```python
from build123d import *

# Parameters (mm, degrees)
BOSS_EXTRUDE1_DEPTH = 25
SKETCH5_R           = 8
BOSS_EXTRUDE2_DEPTH = 35
SKETCH6_R           = 8
BOSS_EXTRUDE3_DEPTH = 35
CUT_EXTRUDE1_DEPTH  = 35
SKETCH9_R           = 5.1
CUT_EXTRUDE2_DEPTH  = 17
SKETCH10_R          = 5.1
CUT_EXTRUDE3_DEPTH  = 17
SKETCH11_R          = 0.5
CUT_EXTRUDE4_DEPTH  = 49.48192396
CUT_EXTRUDE5_REACH  = 44.001
SKETCH12_R          = 1.6
CUT_EXTRUDE7_DEPTH  = 66.003822587


# Read off the part's stored shape, not the designer's step: Mirror1
with BuildPart() as part:
    # Sketch3 → Boss-Extrude1 (new body)
    with BuildSketch(Plane(origin=(0, 0, 0), x_dir=(-0.9678879191476432, 0.2513821313618881, 0), z_dir=(0, 0, 1))):
        Polygon((-6.013757892, -13.576992157), (13.576992157, -6.013757892), (6.013757892, 13.576992157), (-13.576992157, 6.013757892), align=None)
    extrude(amount=BOSS_EXTRUDE1_DEPTH)

    # Sketch5 → Boss-Extrude2 (add)
    with BuildSketch(Plane(origin=(0, 0, 0), x_dir=(-0.6605627762289513, -0.729230336843708, -0.17854952950795708), z_dir=(0.5774000057119382, -0.6454527352206789, 0.499999999999998))):
        with Locations(Location((0, 0, 0), (0, 0, 168.101929209))):
            Circle(SKETCH5_R)
    extrude(amount=BOSS_EXTRUDE2_DEPTH)

    # Sketch6 → Boss-Extrude3 (add)
    with BuildSketch(Plane(origin=(0, 0, 0), x_dir=(-0.7035639492311271, 0.6172392366079582, 0.3521554970945721), z_dir=(-0.4160720061092846, -0.7595288577349762, 0.499999999999998))):
        with Locations(Location((0, 0, 0), (0, 0, 312.286757046))):
            Circle(SKETCH6_R)
    extrude(amount=BOSS_EXTRUDE3_DEPTH)

    # Sketch8 → Cut-Extrude1 (cut)
    with BuildSketch(Plane(origin=(0, 0, 0), x_dir=(-0.9678879191476432, 0.2513821313618881, 0), z_dir=(0, 0, 1))):
        Polygon((-36.845563498, -70.986857451), (-76.079837432, 33.240527854), (43.363854901, 78.202670298), (82.598128835, -26.024715007), align=None)
    extrude(amount=-CUT_EXTRUDE1_DEPTH, mode=Mode.SUBTRACT)

    # Sketch9 → Cut-Extrude2 (cut)
    with BuildSketch(Plane(origin=(20.2090002, -22.590845733, 17.5), x_dir=(0.6605627762289512, 0.7292303368437081, 0.1785495295079571), z_dir=(0.5774000057119382, -0.6454527352206788, 0.499999999999998))):
        with Locations(Location((0, 0, 0), (0, 0, 348.101929209))):
            Circle(SKETCH9_R)
    extrude(amount=-CUT_EXTRUDE2_DEPTH, mode=Mode.SUBTRACT)

    # Sketch10 → Cut-Extrude3 (cut)
    with BuildSketch(Plane(origin=(-14.562520214, -26.583510021, 17.5), x_dir=(-0.7035639492311272, 0.6172392366079582, 0.352155497094572), z_dir=(-0.41607200610928446, -0.7595288577349761, 0.499999999999998))):
        with Locations(Location((0, 0, 0), (0, 0, 129.311285717))):
            Circle(SKETCH10_R)
    extrude(amount=-CUT_EXTRUDE3_DEPTH, mode=Mode.SUBTRACT)

    # Sketch11 → Cut-Extrude4 (cut, through all)
    with BuildSketch(Plane(origin=(0, 0, 25), x_dir=(0.967887919147643, -0.25138213136188803, 0), z_dir=(0, 0, 1))):
        with BuildLine():
            ThreePointArc((-3.837479182, -9.792532706), (-3.837482303, -9.790766245), (-3.837491664, -9.788999807))
            Line((-3.837491664, -9.788999807), (-4.438726063, -10.021113258))
            Line((-4.438726063, -10.021113258), (-4.670839514, -9.419878859))
            ThreePointArc((-4.670839514, -9.419878859), (-4.541586794, -10.248975564), (-3.837479182, -9.792532706))
        make_face()
        with BuildLine():
            Line((-4.438726063, -10.021113258), (-3.837491664, -9.788999807))
            ThreePointArc((-3.837491664, -9.788999807), (-4.134985421, -9.3353716), (-4.670839514, -9.419878859))
            Line((-4.670839514, -9.419878859), (-4.438726063, -10.021113258))
        make_face()
        with BuildLine():
            Line((9.419878859, -4.670839514), (10.021113258, -4.438726063))
            Line((10.021113258, -4.438726063), (9.788999807, -3.837491664))
            ThreePointArc((9.788999807, -3.837491664), (9.3353716, -4.134985421), (9.419878859, -4.670839514))
        make_face()
        with BuildLine():
            Line((9.788999807, -3.837491664), (10.021113258, -4.438726063))
            Line((10.021113258, -4.438726063), (9.419878859, -4.670839514))
            ThreePointArc((9.419878859, -4.670839514), (9.97096067, -4.804558899), (10.292532706, -4.337479182))
            ThreePointArc((10.292532706, -4.337479182), (10.144834814, -3.982678922), (9.788999807, -3.837491664))
        make_face()
        with Locations((-4.337479182, -9.792532706)):
            Circle(SKETCH11_R)
        with Locations((9.792532706, -4.337479182)):
            Circle(SKETCH11_R)
        Polygon((-4.438726063, -10.021113258), (10.021113258, -4.438726063), (4.438726063, 10.021113258), (-10.021113258, 4.438726063), align=None)
    extrude(amount=-CUT_EXTRUDE4_DEPTH, mode=Mode.SUBTRACT)

    # Sketch12 → Cut-Extrude5 (cut, up to next)
    with BuildSketch(Plane(origin=(1.197799286, -10.431456124, 0), x_dir=(0.07381782244775265, 0.008476183382208579, -0.9972357210832067), z_dir=(-0.11407612251429676, 0.9934720118212205, 0)), mode=Mode.PRIVATE) as cut_extrude5_sk1:
        with Locations(Location((-18.947478701, -1.411754543, 0), (0, 0, 274.261167974))):
            Circle(SKETCH12_R)
    cut_extrude5_tool1 = extrude(cut_extrude5_sk1.sketch, amount=CUT_EXTRUDE5_REACH, mode=Mode.PRIVATE) & part.part
    add(cut_extrude5_tool1.solids().sort_by_distance((1.197799, -10.431456, 19))[0], mode=Mode.SUBTRACT)

    # Mirror1: part across plane


with BuildPart() as part_1:
    add(part.part)
    add(part.part.mirror(Plane.XY))

    # Sketch14 → Cut-Extrude7 (cut, through all)
    with BuildSketch(Plane.XY.offset(25)):
        Polygon((-31.040805359, -8.093851281), (38.274007484, -0.134729143), (36.078976394, 18.981470679), (-33.745248602, 10.963854933), align=None)
    extrude(amount=-CUT_EXTRUDE7_DEPTH, mode=Mode.SUBTRACT)


solid = part_1.part
```
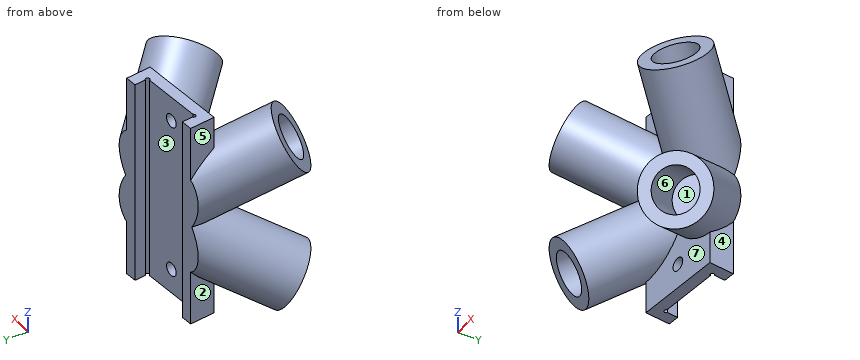
Build history of the part. All positions in model axes, mm. Face numbers are marked on the shaded views. A direction names the side the tool comes from. Round coordinates to 2 decimals unless told otherwise and drop trailing zeros.
Item 1: Pin check, flat tips, straight feed: P1, Ø6, axis at y = -9, z = 9, coming from the +X side; P2, Ø12, axis at y = -25, z = 11, coming from the -X side; P3, Ø1.5, axis at y = -19, z = -17.5, coming from the +X side; P4, Ø10, axis at x = 9.5, y = -17.5, coming from the -Z side. Stop position of each tip, or through.
Item 2: Drill centre lines: line 1 along Z through (x, y) = (-7, -13.75); line 2 along X through (y, z) = (-20.5, 13.5); line 3 along X through (y, z) = (-19.75, 13.5). Where is each one in solid material? Low to high.
Item 3: Saw through at A-A (x = 0.5). State how many separate pieces and enclosed holes the cut face has, then the cut area to 3 significant figures.
Item 4: Two-plate mould, pull along Z, no slides. Class the marked faces 6 and 7: released by +Z, released by -Z, zero draft, split by the parting line, or undercut.
Item 5: Which spindle directions (+Z, -Z, +X, -X, +Y, -Y) get a long thin tool onto all of the face, cutting with end or side? Do the marked faces 1, 2, 3, 4 and 5. Say none if no direction does.
Worked answers:
1. P1: stops at x = 20.73
1. P2: stops at x = -21.84
1. P3: stops at x = 25.28
1. P4: stops at z = -22.61
2. line 1: z = -18.13 to -14.77, -9.29 to 9.29, 14.77 to 18.13
2. line 2: x = -20.03 to -16.84, -5.62 to -2.43, 7.78 to 11.5, 23.11 to 26.01
2. line 3: x = -19.73 to -16.53, -5.35 to -2.16, 7.25 to 10.89, 22.89 to 26.53
3. separate pieces: 3
3. enclosed holes: 0
3. area: 217 mm2
4. face 6: undercut
4. face 7: zero draft
5. face 1: none
5. face 2: -Z, -X
5. face 3: +Z, -Z, +Y
5. face 4: -Z, +X, +Y
5. face 5: +Z, -X
